Input: part model. Units: mm. Frame: model coordinates. A direction names the side the tool comes from. Round coordinates to 2 decimals unless told otherwise and drop trailing zeros. Loops run counter-clockwise (first coordinate to the right, second up) from the corner with the lowest first, then second, coordinate; pieces in that order, holes last. Notation, with made-up numbers: M -39,-27.5 L 17,-27.5 A36 cw 17,7.5 Z; hole C 73,39.25 d10. An arc over 180 degrees is marked long. Use one line per item in the form item = value. Start each with the question number.
Q1. First-contact query: P1, Ø0.6, axis at x = 99, z = 12.5, coming from the +Y side. Flat tip, straight axial feed; report the tip coordinate or a pass-through.
Q2. Mould query, pull axis Y, two halves, no side actions, for faces 1 (the flat face through (112, 7, 10)), 2 (the flat face through (49, 14, 10)), 3 (the flat face through (60, 4, 20)). Classes: pulls with the +Y half, pulls with the -Y half, needs draft (parallel to the pull), parting line crosses it, or undercut.
Q3. Ray query, line 1 along X through (y, z) = (14.75, 11.5); line 2 along Y through (x, z) = (110.5, 13.25); line 3 along Z through (x, y) = (11, 7). Return the intervals inside material, ascending.
Q4. Access query for faces 4 (the flat face through (72, 7, 10)), 5 (the flat face through (80, 12, 10)). Directions: +Z, -Z, +X, -X, +Y, -Y. A direction counts if a zero-diameter tool reaches every point of the face in a straight line with its end or side. Return the directions, or none.
Q5. Section query D-D, the plane y = 3.5. Output: boundary loops of the cut face in (x, z).
Q6. Section query B-B, the plane x = 109.5. Output: boundary loops of the cut face in (y, z), and give its area (3 significant figures).
Q7. Section query A-A, the plane y = 16. Output: boundary loops of the cut face in (x, z), and give its area (3 significant figures).
Q8. Section query C-C, the plane z = 18.5. Output: boundary loops of the cut face in (x, y).
```python
from build123d import *

# Parameters (mm, degrees)
SKETCH1_W           = 18
SKETCH1_H           = 20
BOSS_EXTRUDE1_DEPTH = 20
SKETCH2_W           = 6
SKETCH2_H           = 8
CUT_EXTRUDE1_DEPTH  = 14
SKETCH3_W           = 20
SKETCH3_H           = 5
BOSS_EXTRUDE2_DEPTH = 2
LPATTERN1_COUNT     = 6
LPATTERN1_PITCH     = 20
SKETCH4_W           = 20
SKETCH4_H           = 15
BOSS_EXTRUDE3_DEPTH = 2
SKETCH5_W           = 20
SKETCH5_H           = 20
BOSS_EXTRUDE4_DEPTH = 2
SKETCH7_W           = 106
SKETCH7_H           = 2
CUT_EXTRUDE2_DEPTH  = 2
SKETCH8_W           = 122
SKETCH8_H           = 20
BOSS_EXTRUDE5_DEPTH = 6


with BuildPart() as part:
    # Sketch1 → Boss-Extrude1 (new body)
    with BuildSketch(Plane.XY):
        with Locations((9, 10)):
            Rectangle(SKETCH1_W, SKETCH1_H)
    extrude(amount=BOSS_EXTRUDE1_DEPTH)

    # Sketch2 → Cut-Extrude1 (cut)
    with BuildSketch(Plane.XZ):
        with Locations((9, 10)):
            Rectangle(SKETCH2_W, SKETCH2_H)
    extrude(amount=-CUT_EXTRUDE1_DEPTH, mode=Mode.SUBTRACT)

    # Sketch3 → Boss-Extrude2 (add)
    with BuildSketch(Plane(origin=(18, 0, 0), x_dir=(0, 0, -1), z_dir=(1, 0, 0))):
        with Locations((-10, 2.5)):
            Rectangle(SKETCH3_W, SKETCH3_H)
    extrude(amount=BOSS_EXTRUDE2_DEPTH)


with BuildPart() as lpattern1_1:
    # LPattern1: pattern copy
    add(part.part.moved(Location(Vector(1, 0, 0) * (1 * LPATTERN1_PITCH))))


with BuildPart() as lpattern1_2:
    # LPattern1: pattern copy
    add(part.part.moved(Location(Vector(1, 0, 0) * (2 * LPATTERN1_PITCH))))


with BuildPart() as lpattern1_3:
    # LPattern1: pattern copy
    add(part.part.moved(Location(Vector(1, 0, 0) * (3 * LPATTERN1_PITCH))))


with BuildPart() as lpattern1_4:
    # LPattern1: pattern copy
    add(part.part.moved(Location(Vector(1, 0, 0) * (4 * LPATTERN1_PITCH))))


with BuildPart() as lpattern1_5:
    # LPattern1: pattern copy
    add(part.part.moved(Location(Vector(1, 0, 0) * (5 * LPATTERN1_PITCH))))

    # Sketch4 → Boss-Extrude3 (add)
    with BuildSketch(Plane(origin=(118, 0, 0), x_dir=(0, 0, -1), z_dir=(1, 0, 0))):
        with Locations((-10, 12.5)):
            Rectangle(SKETCH4_W, SKETCH4_H)
    extrude(amount=BOSS_EXTRUDE3_DEPTH)


with BuildPart() as part_1:
    add(part.part)

    # Sketch5 → Boss-Extrude4 (add)
    with BuildSketch(Plane.ZY):
        with Locations((10, 10)):
            Rectangle(SKETCH5_W, SKETCH5_H)
    extrude(amount=BOSS_EXTRUDE4_DEPTH)


with BuildPart() as lpattern1_1_1:
    add(lpattern1_1.part)

    # Combine1: union LPattern1_2, LPattern1_3, LPattern1_4, LPattern1_5, part
    add(lpattern1_2.part)
    add(lpattern1_3.part)
    add(lpattern1_4.part)
    add(lpattern1_5.part)
    add(part_1.part)

    # Sketch7 → Cut-Extrude2 (cut)
    with BuildSketch(Plane(origin=(0, 0, 0), x_dir=(-1, 0, 0), z_dir=(0, -1, 0))):
        with Locations((-59, -10)):
            Rectangle(SKETCH7_W, SKETCH7_H)
    extrude(amount=-CUT_EXTRUDE2_DEPTH, mode=Mode.SUBTRACT)

    # Sketch8 → Boss-Extrude5 (add)
    with BuildSketch(Plane(origin=(0, 0, 0), x_dir=(-1, 0, 0), z_dir=(0, -1, 0))):
        with Locations((-59, -10)):
            Rectangle(SKETCH8_W, SKETCH8_H)
    extrude(amount=BOSS_EXTRUDE5_DEPTH)


solid = lpattern1_1_1.part
```
Results found:
q1.P1 = 5
q2.face_1 = undercut
q2.face_2 = undercut
q2.face_3 = needs draft
q3.line_1 = -2 to 18, 20 to 38, 40 to 58, 60 to 78, 80 to 98, 100 to 120
q3.line_2 = -6 to 0, 14 to 20
q3.line_3 = 0 to 6, 14 to 20
q4.face_4 = none
q4.face_5 = +Z, -Z, +Y
q5.outline = M -2,0 L 120,0 L 120,20 L -2,20 Z; hole M 6,6 L 12,6 L 12,14 L 6,14 Z; hole M 26,6 L 32,6 L 32,14 L 26,14 Z; hole M 46,6 L 52,6 L 52,14 L 46,14 Z; hole M 66,6 L 72,6 L 72,14 L 66,14 Z; hole M 86,6 L 92,6 L 92,14 L 86,14 Z; hole M 106,6 L 112,6 L 112,14 L 106,14 Z
q6.outline = M -6,0 L 20,0 L 20,20 L -6,20 Z; hole M 0,6 L 14,6 L 14,14 L 0,14 Z
q6.area = 408 mm²
q7.outline = M -2,0 L 18,0 L 18,20 L -2,20 Z; M 20,0 L 38,0 L 38,20 L 20,20 Z; M 40,0 L 58,0 L 58,20 L 40,20 Z; M 60,0 L 78,0 L 78,20 L 60,20 Z; M 80,0 L 98,0 L 98,20 L 80,20 Z; M 100,0 L 120,0 L 120,20 L 100,20 Z
q7.area = 2,240 mm²
q8.outline = M -2,-6 L 120,-6 L 120,20 L 100,20 L 100,5 L 98,5 L 98,20 L 80,20 L 80,5 L 78,5 L 78,20 L 60,20 L 60,5 L 58,5 L 58,20 L 40,20 L 40,5 L 38,5 L 38,20 L 20,20 L 20,5 L 18,5 L 18,20 L -2,20 Z
